Input: part model. Units: mm. Frame: model coordinates. Face numbers are marked on the shaded views. A direction names the side the tool comes from. Coordinates: 2 decimals unless noted, no trailing zeros. Write each loop counter-clockwise with the first axis right and the second up, starting at its lowest first coordinate (ties: lowest second). Pieces come first, ordered by that corner, then holes. Notation, with made-up numbers: (44, -8.5) -> (56, -8.5) arc R23 cw to (56, 7.5) -> close; hole circle Ø8 at (74, -20). An arc over 180 degrees is marked (long way). One line per question, with ' | ' between items. Start each with the question number.
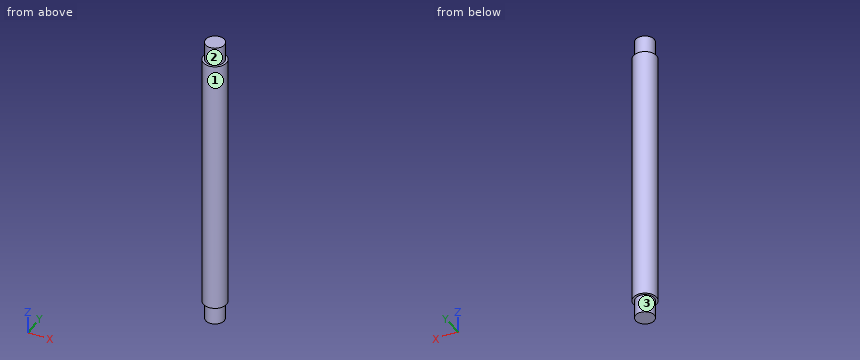
```python
from build123d import *

# Parameters (mm, degrees)
SKETCH1_R           = 5
SKETCH1_R_2         = 4
BOSS_EXTRUDE1_DEPTH = 56.5
SKETCH1_3_R         = 4
BOSS_EXTRUDE2_DEPTH = 64.5


with BuildPart() as part:
    # Sketch1 → Boss-Extrude1 (new, symmetric)
    # profile 1 of 2: a face of its own
    with BuildSketch(Plane.XY):
        Circle(SKETCH1_R)
        Circle(SKETCH1_R_2, mode=Mode.SUBTRACT)
    # profile 2 of 2: a face of its own
    with BuildSketch(Plane.XY):
        Circle(SKETCH1_R_2)
    extrude(amount=BOSS_EXTRUDE1_DEPTH, both=True)

    # Sketch1_3 → Boss-Extrude2 (add, symmetric)
    with BuildSketch(Plane.XY):
        Circle(SKETCH1_3_R)
    extrude(amount=BOSS_EXTRUDE2_DEPTH, both=True)


solid = part.part
```
1) Ray query, line 1 (X direction, y = -0.5, z = -39); line 2 (Y direction, x = 3, z = 17); line 3 (Z direction, x = -2, y = -4). Return the intervals inside material, ascending.
2) Section C-C, the plane z = 50.5. Return loops of the section in (x, y).
3) Section A-A, the plane y = 0. Return loops of the section in (x, z).
4) First-contact query: P1, Ø1, axis at x = -2.5, z = -1.5, coming from the -Y side; P2, Ø2, axis at x = 2, z = 26.5, coming from the +Y side; P3, Ø2, axis at x = 1.5, z = 33, coming from the +Y side; P4, Ø3, axis at x = 3, y = -3.5, coming from the -Z side. Flat tips, straight axial feed; report the tip coordinate or a pass-through.
5) Access query for the marked faces 1, 2 and 3. Directions: +Z, -Z, +X, -X, +Y, -Y. A direction counts if a zero-diameter tool reaches every point of the face in a straight line with its end or side. Return the directions, or none.
Answer block:
1) line 1: x = -4.97 to 4.97 | line 2: y = -4 to 4 | line 3: z = -56.5 to 56.5
2) outline: circle Ø10 at (0, 0)
3) outline: (-5, -56.5) -> (-4, -56.5) -> (-4, -64.5) -> (4, -64.5) -> (4, -56.5) -> (5, -56.5) -> (5, 56.5) -> (4, 56.5) -> (4, 64.5) -> (-4, 64.5) -> (-4, 56.5) -> (-5, 56.5) -> close
4) P1: stops at y = -4.58 | P2: stops at y = 4.9 | P3: stops at y = 4.97 | P4: stops at z = -64.5
5) face 1: +Z, -Z | face 2: +Z | face 3: -Z
